from build123d import *

# Parameters (mm, degrees)
EXTRUDE_1_DEPTH     = 695
SKETCH_2_W          = 695
SKETCH_2_H          = 77.81
EXTRUDE_2_DEPTH     = 50.41
SKETCH_9_W          = 72.82
SKETCH_9_H          = 51.4
CUT_EXTRUDE_3_DEPTH = 1000
SKETCH_10_W         = 72.82
SKETCH_10_H         = 51.4
CUT_EXTRUDE_4_DEPTH = 1000


with BuildPart() as part:
    # 草图1 → 凸台-拉伸1 (new body)
    with BuildSketch(Plane(origin=(0, 0, 0), x_dir=(0, 0, -1), z_dir=(1, 0, 0))):
        Polygon((51.711180709, 31.822265051), (-12.508819291, 31.822265051), (-12.508819291, -45.987734949), align=None)
    extrude(amount=EXTRUDE_1_DEPTH)

    # 草图2 → 凸台-拉伸2 (add)
    with BuildSketch(Plane.XY.offset(12.508819291)):
        with Locations((347.5, -7.082734949)):
            Rectangle(SKETCH_2_W, SKETCH_2_H)
    extrude(amount=EXTRUDE_2_DEPTH)

    # 草图9 → 切除-拉伸3 (cut)
    with BuildSketch(Plane(origin=(0, 31.822265051, 0), x_dir=(1, 0, 0), z_dir=(0, 1, 0))):
        with Locations((63.6, -37.218819291)):
            Rectangle(SKETCH_9_W, SKETCH_9_H)
    extrude(amount=-CUT_EXTRUDE_3_DEPTH, mode=Mode.SUBTRACT)

    # 草图10 → 切除-拉伸4 (cut)
    with BuildSketch(Plane(origin=(0, 31.822265051, 0), x_dir=(1, 0, 0), z_dir=(0, 1, 0))):
        with Locations((631.4, -37.218819291)):
            Rectangle(SKETCH_10_W, SKETCH_10_H)
    extrude(amount=-CUT_EXTRUDE_4_DEPTH, mode=Mode.SUBTRACT)


solid = part.part
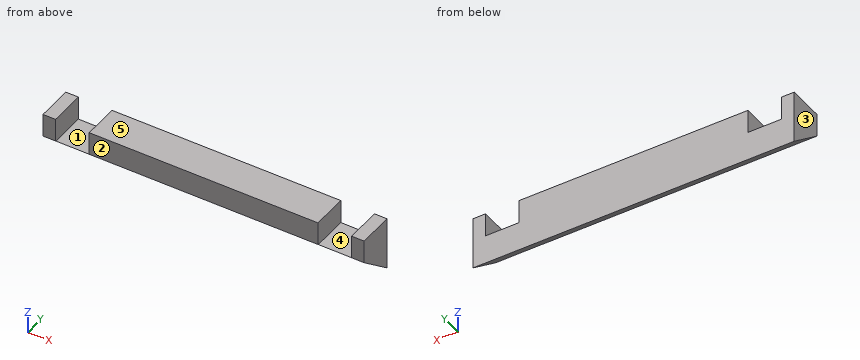
CAD build for the part. Positions are in the model's coordinates, mm. Face numbers are marked on the shaded views. A direction names the side the tool comes from. Give positions to 0.01 mm unless a question says otherwise; leave off trailing zeros. Order: outer loops, then holes, each group sorted by start corner. A loop starts at its lowest first (then second) coordinate and runs counter-clockwise, first axis right, second up. Notation, with made-up numbers: (25.25, 59.25) - (70.25, 59.25) arc R16 ccw to (70.25, 69.25) - close; hole circle Ø3 at (86.25, 85.25). An arc over 180 degrees is marked (long way). Write each question's results on one line, items separated by ' | '.
1. Saw through at D-D on y = 0.5. List the corners of the cut face in (x, z).
Calculated:
outline: (0, -25.86) - (695, -25.86) - (695, 62.92) - (667.81, 62.92) - (667.81, 11.52) - (594.99, 11.52) - (594.99, 62.92) - (100.01, 62.92) - (100.01, 11.52) - (27.19, 11.52) - (27.19, 62.92) - (0, 62.92) - close
2. Saw through at C-C on x = 43. List the corners of the cut face in (y, z), and give its area (3 significant figures).
Calculated:
outline: (-44.79, 11.52) - (31.82, -51.71) - (31.82, 11.52) - close | area: 2,420 mm2
3. Saw through at B-B on y = -26. List the corners of the cut face in (x, z), and give its area (3 significant figures).
Calculated:
outline: (0, -3.99) - (695, -3.99) - (695, 62.92) - (667.81, 62.92) - (667.81, 11.52) - (594.99, 11.52) - (594.99, 62.92) - (100.01, 62.92) - (100.01, 11.52) - (27.19, 11.52) - (27.19, 62.92) - (0, 62.92) - close | area: 39,000 mm2
4. 3-axis set-ups, long thin cutter, end or side, ignore diameter. For the marked faces 1 and 2: which of +Z, -Z, +X, -X, +Y, -Y reach the whole face in a straight line?
Calculated:
face 1: +Z, +Y, -Y | face 2: +Z, -Z, +X, -X, -Y
5. Pull direction X, two halves, no side cores. Call the marked faces 3, 4 and 5: released by +X, released by -X, zero draft, split by the parting line, or undercut.
Calculated:
face 3: released by -X | face 4: undercut | face 5: zero draft
6. Saw through at A-A on z = 28.5. List the corners of the cut face in (x, y), and give its area (3 significant figures).
Calculated:
outline: (0, -45.99) - (27.19, -45.99) - (27.19, 31.82) - (0, 31.82) - close; (100.01, -45.99) - (594.99, -45.99) - (594.99, 31.82) - (100.01, 31.82) - close; (667.81, -45.99) - (695, -45.99) - (695, 31.82) - (667.81, 31.82) - close | area: 42,700 mm2
7. Probe L1, parallel to X at y = -13.5, z = 33; L2, parallel to Z at x = 136, y = 25; L3, parallel to Y at x = 592, z = -4. List the from-to ranges inside material, lowest first. Write a range as from..to.
Calculated:
L1: x = 0..27.19, 100.01..594.99, 667.81..695 | L2: z = -46.08..62.92 | L3: y = -25.99..31.82
8. Pin check, flat tips, straight feed: pin 1 (8 mm diameter, centred on x = 78.5, y = 19, fed in from -Z); pin 2 (2 mm diameter, centred on x = 158, y = -7.5, fed in from -Z); pin 3 (4 mm diameter, centred on x = 559, y = 12.5, fed in from -Z). Stop position of each tip, or through.
Calculated:
pin 1: stops at z = -44.43 | pin 2: stops at z = -20.08 | pin 3: stops at z = -37.41
